Verification items for the finished model (mm, model axes). A direction names the side the tool comes from. Coordinates: 2 decimals unless noted, no trailing zeros. Loops run counter-clockwise (first coordinate to the right, second up) from the corner with the lowest first, then second, coordinate; pieces in that order, holes last. Notation, with made-up numbers: (-38.75, 8) -> (-0.75, 8) arc R26 cw to (-0.75, 29) -> close; hole circle Ø3 at (50.5, 68.5). An arc over 180 degrees is marked (long way). Write item = value, one per line.
Autodesk Inventor part; units mm, degrees
ref_plane "YZ Plane" through (0, 0, 0) normal (1, 0, 0) x (0, 1, 0)
ref_plane "XZ Plane" through (0, 0, 0) normal (0, 1, 0) x (-1, 0, 0)
ref_plane "XY Plane" through (0, 0, 0) normal (0, 0, 1) x (1, 0, 0)
sketch "Sketch1" plane through (0, 0, 0) normal (0, 0, 1) x (1, 0, 0)
  line L0 (0, 0) -> (101.6, 0)
  line L1 (101.6, 0) -> (101.6, 53.975)
  line L2 (101.6, 53.975) -> (0, 53.975)
  line L3 (0, 53.975) -> (0, 0)
  circle A0 centre (50.8, 28.575) radius 14.2875
  line L4 (23.8125, 28.575) -> (50.8, 28.575) construction
  line L5 (50.8, 28.575) -> (77.7875, 28.575) construction
  line L6 (50.8, 28.575) -> (50.8, 53.975) construction
  line L7 (101.6, 0) -> (101.6, -6.35)
  line L8 (101.6, -6.35) -> (0, -6.35)
  line L9 (0, -6.35) -> (0, 0)
  line L10 (0, 53.975) -> (101.6, 53.975)
  line L11 (101.6, 53.975) -> (101.6, 60.325)
  line L12 (101.6, 60.325) -> (0, 60.325)
  line L13 (0, 60.325) -> (0, 53.975)
  point P0 (9.704, 43.7695)
  point P1 (91.896, 43.7695)
  dimension "d0" = 53.975
  dimension "d2" = 101.6
  dimension "d3" = 28.575
  dimension "d4" = 50.8
  dimension "d5" = 28.575
  dimension "d6" = 26.9875
  dimension "d7" = 41.096
  dimension "d8" = 15.1945
  dimension "d9" = 6.35
  dimension "d10" = 6.35
extrude "Extrusion1" add sketch "Sketch1" along normal blind 6.35
extrude "Extrusion2" cut sketch "Sketch1" along normal blind 3.175 contours L3 L2 L1 L0
hole "Hole1" at (23.8125, 28.575, 0) at (77.7875, 28.575, 0) direction (0, 0, 1) diameter 6.35 end through all
hole "Hole2" at (9.704, 43.7695, 0) at (91.896, 43.7695, 0) direction (0, 0, 1) diameter 9.525 end through all
equation "\"d4\" = 0.5 * d2"
properties part number "Mounting Jig"
1) Sectioned sample at C-C, the plane y = 44.5. Record the cut outline in (x, z) (3 decimals), plus the area to 3 significant figures.
Ans:
outline = (0, 3.175) -> (4.998, 3.175) -> (4.998, 6.35) -> (0, 6.35) -> close; (14.41, 3.175) -> (87.19, 3.175) -> (87.19, 6.35) -> (14.41, 6.35) -> close; (96.602, 3.175) -> (101.6, 3.175) -> (101.6, 6.35) -> (96.602, 6.35) -> close
area = 263 mm2
2) Depth check by flat-ended pin: pin 1 Ø5.5 at (x, y) = (9.7, 43.77) entering from +Z; pin 2 Ø8.5 at (x, y) = (77.79, 28.58) entering from -Z (3 decimals). Enter the tip coordinate at first touch or a pass-through.
Ans:
pin_1 = through
pin_2 = 3.175
3) Sectioned sample at D-D, the plane x = 93.5. Record the cut outline in (y, z) (3 decimals).
Ans:
outline = (-6.35, 0) -> (0, 0) -> (0, 3.175) -> (39.285, 3.175) -> (39.285, 6.35) -> (-6.35, 6.35) -> close; (48.254, 3.175) -> (53.975, 3.175) -> (53.975, 0) -> (60.325, 0) -> (60.325, 6.35) -> (48.254, 6.35) -> close
4) Material ranges on line 1 (Y direction, x = 76, z = 2.5) (3 decimals); line 2 (Z direction, x = 46.5, y = 50.5) (3 decimals); line 3 (Y direction, x = 8.5, z = 3.5) (3 decimals), recorded low to high.
Ans:
line_1 = -6.35 to 0, 53.975 to 60.325
line_2 = 3.175 to 6.35
line_3 = -6.35 to 39.162, 48.377 to 60.325
5) Sectioned sample at A-A, the plane z = 1.5. Record the cut outline in (x, y) (3 decimals), plus the area to 3 significant figures.
Ans:
outline = (0, -6.35) -> (101.6, -6.35) -> (101.6, 0) -> (0, 0) -> close; (0, 53.975) -> (101.6, 53.975) -> (101.6, 60.325) -> (0, 60.325) -> close
area = 1,290 mm2
6) Tool access check on faces 1 (the face through (50, 0, 2)), 2 (the face through (101.6, 27, 5)). Record the directions out of +Z, -Z, +X, -X, +Y, -Y that give a thin tool (end or side, any length) a straight path to the whole face; none if there is none.
Ans:
face_1 = -Z, +X, -X
face_2 = +Z, -Z, +X, +Y, -Y
7) Release check for a two-part mould opening along X. For faces 3 (the face through (0, 27, 5)), 4 (the face through (52, 60.325, 3)), 5 (the face through (4.98, 43.15, 4.78)) record: pulls with the +X half, pulls with the -X half, needs draft (parallel to the pull), parting line crosses it, or undercut.
Ans:
face_3 = pulls with the -X half
face_4 = needs draft
face_5 = undercut
